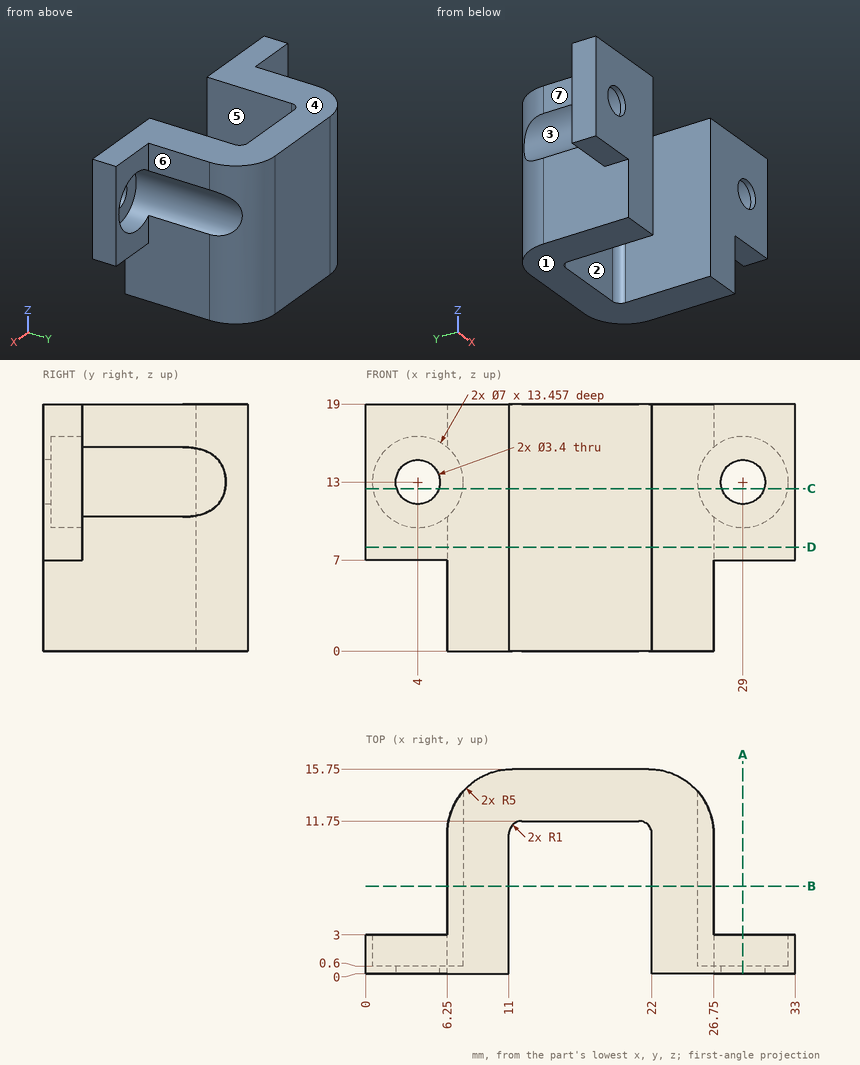
Geometry check sheet. Reference: drawing and pictorial views, mm from the part's lowest x, y, z. A direction names the side the tool comes from. Give positions to 0.01 mm unless a question says otherwise; leave off trailing zeros. Order: outer loops, then holes, each group sorted by start corner. A loop starts at its lowest first (then second) coordinate and runs counter-clockwise, first axis right, second up. Notation, with made-up numbers: M -21,-29.5 L -16,-29.5 A17 cw -16,-1.5 Z; hole C 89.25,-1.5 d9. An arc over 180 degrees is marked long. Answer in a Markdown table with one row per item. Add a question column.
Item 1: Mould release check, pull along Z, two halves, no side actions. Record for the marked faces 1, 2, 3 and 4: released by +Z, released by -Z, zero draft, split by the parting line, or undercut.
Item 2: Section check A-A, the plane x = 29. Enter the section's corners in (y, z).
Item 3: Section check C-C, the plane z = 12.5. State how many separate pieces and enclosed holes the cut face has, and give its area (3 significant figures).
Item 4: Tool access check on the marked faces 5, 6 and 7. Record the directions out of +Z, -Z, +X, -X, +Y, -Y that give a thin tool (end or side, any length) a straight path to the whole face; none if there is none.
Item 5: Scan lines: probe 1 along X at (y, z) = (8.25, 16.5); probe 2 along X at (y, z) = (1.5, 10). Record each from-to range of solid material in increasing order. Write a range as from..to.
Item 6: Gauge pin test, flat ends, axial feed: pin 1 (4 mm diameter, centred on x = 4, z = 13, fed in from +Y); pin 2 (1.7 mm diameter, centred on y = 7, z = 17, fed in from -X); pin 3 (7 mm diameter, centred on x = 29, z = 14.5, fed in from +Y); pin 4 (2 mm diameter, centred on x = 29, z = 13, fed in from -Y). Record the tip position at first contact, or that the pin passes through.
Item 7: Section check B-B, the plane y = 6.75. Enter the section's corners in (x, z), and give its area (3 significant figures).
Item 8: Section check D-D, the plane z = 8. Enter the section's corners in (x, y), and give its area (3 significant figures).
Filled sheet:
| question | item | result |
|---|---|---|
| 1 | face 1 | released by -Z |
| 1 | face 2 | zero draft |
| 1 | face 3 | undercut |
| 1 | face 4 | released by +Z |
| 2 | outline | M 0,7 L 3,7 L 3,9.5 L 0.6,9.5 L 0.6,11.3 L 0,11.3 Z; M 0,14.7 L 0.6,14.7 L 0.6,16.5 L 3,16.5 L 3,19 L 0,19 Z |
| 3 | separate pieces | 3 |
| 3 | enclosed holes | 0 |
| 3 | area | 159 mm^2 |
| 4 | face 5 | +Z, -Z, -Y |
| 4 | face 6 | +Z, -Z, +X, +Y |
| 4 | face 7 | +Z, -Z, -X, +Y |
| 5 | probe 1 | x = 6.25..11, 22..26.75 |
| 5 | probe 2 | x = 0..2.2, 5.8..11, 22..27.2, 30.8..33 |
| 6 | pin 1 | stops at y = 0.6 |
| 6 | pin 2 | stops at x = 6.25 |
| 6 | pin 3 | stops at y = 14.06 |
| 6 | pin 4 | passes through |
| 7 | outline | M 6.25,0 L 11,0 L 11,19 L 6.25,19 L 6.25,15.68 A3.5 cw 6.25,10.32 Z; M 22,0 L 26.75,0 L 26.75,10.32 A3.5 cw 26.75,15.68 L 26.75,19 L 22,19 Z |
| 7 | area | 171 mm^2 |
| 8 | outline | M 0,0 L 11,0 L 11,10.75 A1 cw 12,11.75 L 21,11.75 A1 cw 22,10.75 L 22,0 L 33,0 L 33,3 L 26.75,3 L 26.75,10.75 A5 ccw 21.75,15.75 L 11.25,15.75 A5 ccw 6.25,10.75 L 6.25,3 L 0,3 Z |
| 8 | area | 221 mm^2 |
